For this review, take the finished solid that the model builds, in its own axes (mm). A direction names the side the tool comes from. Coordinates: 2 decimals unless noted, no trailing zeros. Order: outer loops, then holes, each group sorted by start corner. A loop starts at its lowest first (then second) coordinate and runs counter-clockwise, first axis right, second up. Notation, with made-up numbers: (53.5, 59) -> (104.5, 59) arc R14 cw to (104.5, 75) -> close; hole circle Ø1 at (-29, 49). An arc over 180 degrees is marked (long way). Write item = value, one per line. Start each with the question number.
1) Consider section C-C on z = -2.25. Give the boundary of the cut face in (x, y).
2) Consider section B-B on x = 0. Give the boundary of the cut face in (y, z).
3) Consider section A-A on y = 0. Give the boundary of the cut face in (x, z).
4) Machinability: for faces 4 (the face through (1.853, -7.441, -3.042)), 5 (the face through (0, 8.043, -3)), 6 (the face through (0, -8.043, -3)), which of the approach directions +Z, -Z, +X, -X, +Y, -Y give a long, thin tool a straight path to every point of the face, cutting with its end or side? Answer none if there is none.
5) Consider section D-D on z = 11.75. Give the boundary of the cut face in (x, y).
6) Draft analysis for pull direction Y (two halves, no side actions). For faces 1 (the face through (-1.822, 7.473, -3.042)), 2 (the face through (-1.853, -7.441, -3.042)), 3 (the face through (0, 0, -3.86)), state which applies: +Y half, -Y half, draft (parallel to the pull), parting line (faces both ways), or undercut.
7) Insertion check: pin 1 Ø5 at (y, z) = (0, -3.5) entering from -X; pin 2 Ø1.5 at (y, z) = (4.5, 4) entering from -X; pin 3 Ø2 at (x, z) = (-1, -2.5) entering from +Y. Each pin has a flat end and moves straight along its axis. Give the tip position at first contact, or say it passes through.
8) Wall thickness on probe 1 along Z at (x, y) = (0.25, -0.75); probe 2 along Z at (x, y) = (3.25, 2.75); probe 3 along X at (y, z) = (1, -1.5): over which ranges is each line inside the solid? List them lowest first. Write a range as [from, to].
from build123d import *

# Parameters (mm, degrees)
SKETCH_1_R          = 8.4
EXTRUDE_1_DEPTH     = 10
SKETCH_2_R          = 7.5
EXTRUDE_2_DEPTH     = 10
EXTRUDE_2_TAPER     = 3.0000000000000027
SKETCH_3_W          = 4.846227442126801
SKETCH_3_H          = 16.08583474921887
EXTRUDE_3_DEPTH     = 6
FILLET_1_R          = 2
FILLET_2_R          = 1
CUT_EXTRUDE_1_DEPTH = 25.24252038183517


with BuildPart() as part:
    # Эскиз1 → Бобышка-Вытянуть1 (new body)
    with BuildSketch(Plane.XY):
        Circle(SKETCH_1_R)
    extrude(amount=EXTRUDE_1_DEPTH)

    # Эскиз2 → Бобышка-Вытянуть2 (add)
    with BuildSketch(Plane.XY.offset(10)):
        Circle(SKETCH_2_R)
    extrude(amount=EXTRUDE_2_DEPTH, taper=EXTRUDE_2_TAPER)

    # Эскиз3 → Бобышка-Вытянуть3 (add)
    with BuildSketch(Plane(origin=(0, 0, 0), x_dir=(-1, 0, 0), z_dir=(0, 0, -1))):
        Rectangle(SKETCH_3_W, SKETCH_3_H)
    extrude(amount=EXTRUDE_3_DEPTH)

    # Скругление1
    fillet_1_edges = [part.edges().sort_by_distance(p)[0] for p in [
        (-2.4231137210634004, -8.042917374609434, -3),
        (-2.4231137210634004, 8.042917374609434, -3),
        (2.4231137210634004, 8.042917374609434, -3),
        (2.4231137210634004, -8.042917374609434, -3),
    ]]
    fillet(fillet_1_edges, radius=FILLET_1_R)

    # Скругление2
    # the kernel refuses this fillet: 1 mm, written as the material it adds along each edge
    with BuildSketch(Plane(origin=(-6.3e-16, 6.7e-16, 10), x_dir=(1, -3.3e-16, 0), z_dir=(3.3e-16, 1, 0))) as fillet_2_piece_1:
        with BuildLine():
            CenterArc((8.449027591022826, -0.9987974245654119), FILLET_2_R, 92.81020062838743, 84.18979937161257)
            Line((7.450398056268253, -0.9464614683224681), (7.430425465573162, -0.9454147491976084))
            Line((7.430425465573162, -0.9454147491976084), (7.48002740930491, 0.00104671912485976))
            Line((7.48002740930491, 0.00104671912485976), (7.500000000000001, 0.01999999999999957))
            ThreePointArc((7.500000000000001, 0.01999999999999957), (7.950000000000001, 0.01999999999999957), (8.399019448179544, 0.01997594849130735))
            Line((8.399019448179544, 0.01997594849130735), (8.4, 0))
        make_face()
    revolve(axis=Axis((-6.3e-16, 6.7e-16, 10), (0, 0, -1)))

    # Эскиз4 → Вырез-Вытянуть1 (cut, through all)
    with BuildSketch(Plane.ZY.offset(2.4231137210634004)):
        Polygon((-3.85980947138648, 3.9999999999999982), (-1.85980947138648, 3.9999999999999982), (-1.8598094713864777, -4.000000000000001), (-3.85980947138648, -4.000000000000002), align=None)
    extrude(amount=-CUT_EXTRUDE_1_DEPTH, mode=Mode.SUBTRACT)


solid = part.part
Answer sheet:
q1.outline = (-2.42, -6.04) arc R2 ccw to (-0.42, -8.04) -> (0.42, -8.04) arc R2 ccw to (2.42, -6.04) -> (2.42, -4) -> (-2.42, -4) -> close; (-2.42, 4) -> (2.42, 4) -> (2.42, 6.04) arc R2 ccw to (0.42, 8.04) -> (-0.42, 8.04) arc R2 ccw to (-2.42, 6.04) -> close
q2.outline = (-8.4, 0) -> (-8.04, 0) -> (-8.04, -6) -> (8.04, -6) -> (8.04, 0) -> (8.4, 0) -> (8.4, 10) arc R1 cw to (7.45, 10.95) -> (6.98, 20) -> (-6.98, 20) -> (-7.45, 10.95) arc R1 cw to (-8.4, 10) -> close; hole (-4, -3.86) -> (4, -3.86) -> (4, -1.86) -> (-4, -1.86) -> close
q3.outline = (-8.4, 0) -> (-2.42, 0) -> (-2.42, -1.86) -> (2.42, -1.86) -> (2.42, 0) -> (8.4, 0) -> (8.4, 10) arc R1 cw to (7.45, 10.95) -> (6.98, 20) -> (-6.98, 20) -> (-7.45, 10.95) arc R1 cw to (-8.4, 10) -> close; (-2.42, -6) -> (2.42, -6) -> (2.42, -3.86) -> (-2.42, -3.86) -> close
q4.face_4 = -Z, +X, -Y
q4.face_5 = -Z, +X, -X, +Y
q4.face_6 = -Z, +X, -X, -Y
q5.outline = circle Ø14.82 at (0, 0)
q6.face_1 = +Y half
q6.face_2 = -Y half
q6.face_3 = undercut
q7.pin_1 = -2.42
q7.pin_2 = -7.52
q7.pin_3 = 8.04
q8.probe_1 = [-6, -3.86], [-1.86, 20]
q8.probe_2 = [0, 20]
q8.probe_3 = [-2.42, 2.42]
